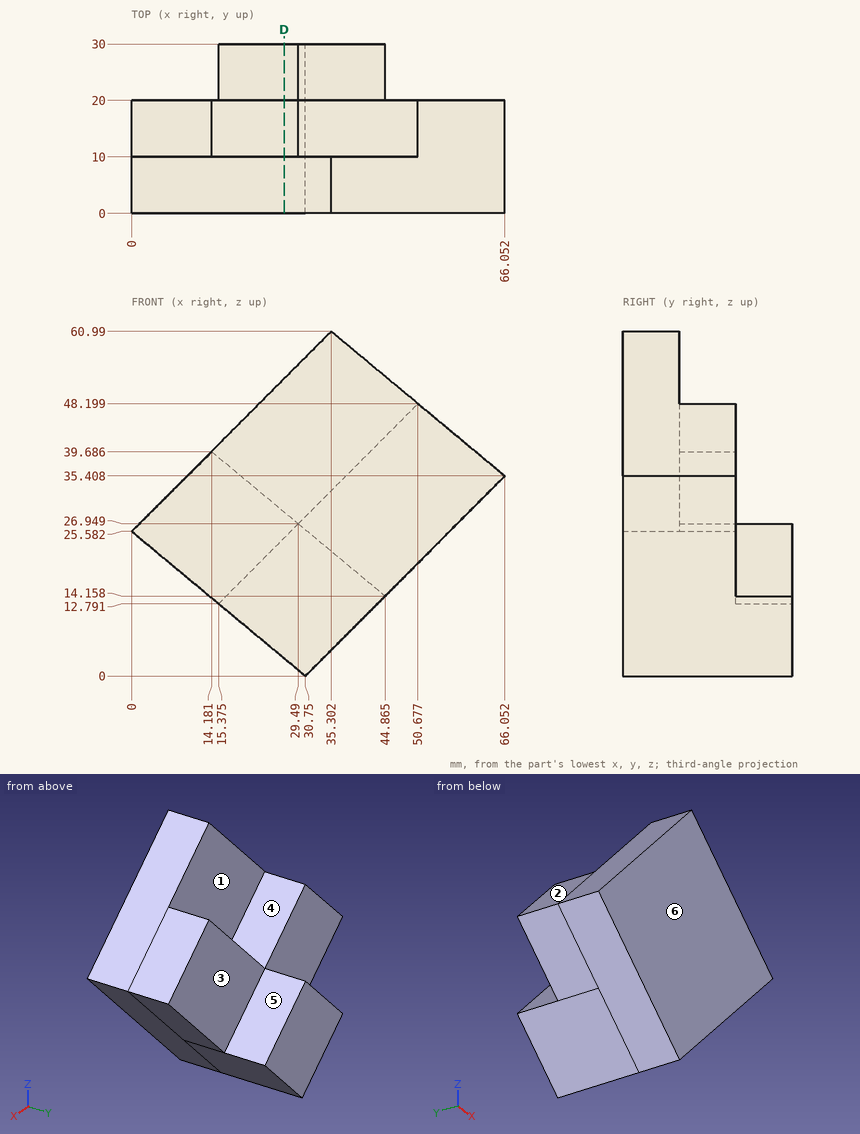
Drawing for the job (mm, zero at the part's lowest x, y, z). A direction names the side the tool comes from. Round coordinates to 2 decimals unless told otherwise and drop trailing zeros. Loops run counter-clockwise (first coordinate to the right, second up) from the corner with the lowest first, then second, coordinate; pieces in that order, holes last.
1. Wall check: probe 1 along Y at (x, z) = (6.5, 27); probe 2 along X at (y, z) = (9.75, 55) (1 decimal); probe 3 along X at (y, z) = (17.5, 14) (1 decimal). Give the ranges that are in metal, low to high.
Check values:
probe 1: y = 0 to 20
probe 2: x = 29.3 to 42.5
probe 3: x = 13.9 to 44.7
2. Drop flat-ended pins along their axis: P1, Ø2, axis at x = 30, y = 10.5, coming from the +Z side; P2, Ø1, axis at y = 15.5, z = 17.5, coming from the -X side (1 decimal); P3, Ø6, axis at x = 59, y = 24, coming from the +Z side; P4, Ø21.5, axis at x = 9.5, z = 28, coming from the +Y side. Give the stop position or say it passes through.
Check values:
P1: stops at z = 56.54
P2: stops at x = 9.1
P3: passes through
P4: stops at y = 20
3. Tool access for the marked faces 1, 2 and 3: list every direction of +Z, -Z, +X, -X, +Y, -Y with a clear straight run to the whole face (end or side of a thin tool).
Check values:
face 1: +Z, +Y
face 2: +Z, -X, +Y
face 3: +Z, +X, +Y
4. Mould opens along X. For the marked faces 4, 5 and 6 say: +X half, -X half, draft (parallel to the pull), parting line (faces both ways), or undercut.
Check values:
face 4: undercut
face 5: +X half
face 6: draft
5. Band-saw the part on D-D, the plane x = 27. List the corners of the cut face in (y, z).
Check values:
outline: (0, 3.12) - (30, 3.12) - (30, 24.45) - (20, 24.45) - (20, 29.02) - (10, 29.02) - (10, 52.66) - (0, 52.66) - close
